from build123d import *

# Parameters (mm, degrees)
SKETCH1_R                     = 55
BOSS_EXTRUDE1_DEPTH           = 10
SKETCH6_R                     = 50
BOSS_EXTRUDE3_DEPTH           = 5
SKETCH9_R                     = 2
CUT_EXTRUDE2_DEPTH            = 8
BOSS_EXTRUDE4_START           = -5
SKETCH24_R                    = 60
SKETCH24_R_2                  = 55
BOSS_EXTRUDE4_DEPTH           = 5
CBORE_FOR_M3_SHCS1_AT_2_COUNT = 2
CBORE_FOR_M3_SHCS1_AT_2_PITCH = 70
CBORE_FOR_M3_SHCS1_AT_3_COUNT = 2
CBORE_FOR_M3_SHCS1_AT_3_PITCH = 70
CBORE_FOR_M3_SHCS1_AT_4_COUNT = 2
CBORE_FOR_M3_SHCS1_AT_4_PITCH = 98.994949366
CHAMFER2_SIZE                 = 1


with BuildPart() as part:
    # Sketch1 → Boss-Extrude1 (new body)
    with BuildSketch(Plane.XY):
        Circle(SKETCH1_R)
    extrude(amount=-BOSS_EXTRUDE1_DEPTH)

    # Sketch6 → Boss-Extrude3 (add)
    with BuildSketch(Plane(origin=(0, 0, -10), x_dir=(-1, 0, 0), z_dir=(0, 0, -1))):
        Circle(SKETCH6_R)
    extrude(amount=-BOSS_EXTRUDE3_DEPTH)

    # Sketch9 → Cut-Extrude2 (cut)
    with BuildSketch(Plane.XY):
        with Locations((23.676144844, -19.05)):
            Circle(SKETCH9_R)
        with Locations((-24.583855156, -17.78)):
            Circle(SKETCH9_R)
        with Locations((18.596144844, 33.02)):
            Circle(SKETCH9_R)
        with Locations((-9.343855156, 33.02)):
            Circle(SKETCH9_R)
    extrude(amount=-CUT_EXTRUDE2_DEPTH, mode=Mode.SUBTRACT)

    # Sketch24 → Boss-Extrude4 (add)
    with BuildSketch(Plane(origin=(0, 0, -10), x_dir=(-1, 0, 0), z_dir=(0, 0, -1)).offset(BOSS_EXTRUDE4_START)):
        Circle(SKETCH24_R)
        with Locations(Location((0, 0, 0), (0, 0, 180))):
            Circle(SKETCH24_R_2, mode=Mode.SUBTRACT)
    extrude(amount=BOSS_EXTRUDE4_DEPTH)

    # Sketch26 → CBORE for M3 SHCS1 (revolve, cut)
    with BuildSketch(Plane(origin=(-35, -35, -10), x_dir=(0, 1, 0), z_dir=(1, 0, 0))):
        Polygon((0, 0), (0, 10), (1.7, 10), (1.7, 3), (3.25, 3), (3.25, 0.025), (3.275, 0), align=None)
    cbore_for_m3_shcs1 = revolve(axis=Axis((-35, -35, -16.35), (0, 0, 1)), mode=Mode.SUBTRACT)

    # CBORE for M3 SHCS1 at 2: CBORE for M3 SHCS1 ×2
    with Locations(*[(0, i * CBORE_FOR_M3_SHCS1_AT_2_PITCH, 0) for i in range(1, CBORE_FOR_M3_SHCS1_AT_2_COUNT)]):
        add(cbore_for_m3_shcs1, mode=Mode.SUBTRACT)

    # CBORE for M3 SHCS1 at 3: CBORE for M3 SHCS1 ×2
    with Locations(*[(i * CBORE_FOR_M3_SHCS1_AT_3_PITCH, 0, 0) for i in range(1, CBORE_FOR_M3_SHCS1_AT_3_COUNT)]):
        add(cbore_for_m3_shcs1, mode=Mode.SUBTRACT)

    # CBORE for M3 SHCS1 at 4: CBORE for M3 SHCS1 ×2
    with Locations(*[Vector(0.7071067811865476, 0.7071067811865476, 0) * (i * CBORE_FOR_M3_SHCS1_AT_4_PITCH) for i in range(1, CBORE_FOR_M3_SHCS1_AT_4_COUNT)]):
        add(cbore_for_m3_shcs1, mode=Mode.SUBTRACT)

    # Chamfer2
    chamfer2_edges = [part.edges().sort_by_distance(p)[0] for p in [
        (-55, 0, 0),
    ]]
    chamfer(chamfer2_edges, length=CHAMFER2_SIZE)


solid = part.part
The model under review builds one solid part; all positions refer to its coordinate system, in mm. A direction names the side the tool comes from. Round coordinates to 2 decimals unless told otherwise and drop trailing zeros. Write each loop counter-clockwise with the first axis right and the second up, starting at its lowest first coordinate (ties: lowest second). Pieces come first, ordered by that corner, then holes. Notation, with made-up numbers: M 35,2 L 92,2 A32 ccw 92,30 Z; hole C -23.5,-16.75 d8. An arc over 180 degrees is marked long. Answer as CSV lines item,"result". Start each with the question number.
Q1. Wall thickness on line 1 along X through (y, z) = (-35, -9.05); line 2 along Y through (x, z) = (-35, -3); line 3 along Z through (x, y) = (37, 47): over which ranges is each line inside the solid? List them lowest first.
Q2. Clearance check with flat-ended pins moving along their axes: P1, Ø6, axis at x = 8.5, z = -7, coming from the +Y side; P2, Ø4.5, axis at x = 35, y = -35, coming from the -Z side; P3, Ø2, axis at y = 43.5, z = -1, coming from the +X side; P4, Ø2, axis at x = 35, y = 35, coming from the +Z side. State where each tip first meets the part, or that it passes through.
Q3. Tool access review of faces 4 (the face through (-9, 33, -8)), 5 (the face through (-32.117, 36.5, -8.508)), 6 (the face through (-1, 1, 0)): name each direction out of +Z, -Z, +X, -X, +Y, -Y from which nothing blocks a thin tool from reaching the whole face with its end or side.
Q4. The part is to be moulded in two halves that separate along Y. For faces 1 (the face through (-33.34, -35.37, -3.55)), 2 (the face through (-11.923, -53.692, -2.972)), 3 (the face through (-26, -49, -5)), say which applies: +Y half, -Y half, draft (parallel to the pull), parting line (faces both ways), or undercut.
Q5. Consider section A-A, the plane y = 0. Give the boundary of the cut face in (x, z), then the cut area to 3 significant figures.
Q6. Consider section C-C, the plane x = -35. State how many separate pieces and enclosed holes the cut face has, then the cut area to 3 significant figures.
Result set:
1,line 1,"x = -48.73 to -38.25, -31.75 to 31.75, 38.25 to 48.73"
1,line 2,"y = -42.43 to -36.7, -33.3 to 33.3, 36.7 to 42.43"
1,line 3,"z = -10 to -5"
2,P1,"stops at y = 59.75"
2,P2,"stops at z = -7"
2,P3,"stops at x = 34.91"
2,P4,"passes through"
3,face 4,"+Z"
3,face 5,"-Z"
3,face 6,"+Z, +X, -X, +Y, -Y"
4,face 1,"undercut"
4,face 2,"parting line"
4,face 3,"draft"
5,outline,"M -60,-10 L 60,-10 L 60,-5 L 55,-5 L 55,-1 L 54,0 L -54,0 L -55,-1 L -55,-5 L -60,-5 Z"
5,area,"1,150 mm²"
6,separate pieces,"3"
6,enclosed holes,"0"
6,area,"824 mm²"
